Here's how the part is built. I have some questions about the finished solid (model axes, mm). A direction names the side the tool comes from. Round coordinates to 2 decimals unless told otherwise and drop trailing zeros. Write each loop counter-clockwise with the first axis right and the second up, starting at its lowest first coordinate (ties: lowest second). Pieces come first, ordered by that corner, then holes. Notation, with made-up numbers: (5.25, -21.5) - (43.25, -21.5) arc R20 ccw to (43.25, -11.5) - close; hole circle Ø7 at (40, 29). An arc over 180 degrees is marked (long way). Write item = value, one per line. Start each with the question number.
Item 1: If we section it at D-D (z = -11.25): Give the number of separate pieces and of enclosed holes in the cut face, and give its area (3 significant figures).
Item 2: If we section it at C-C (y = 16): Please give me the cut outline in (x, z).
Item 3: Thinking about a two-plate mould opening in Y: for faces 1 (the face through (-13, 66, -4)), 2 (the face through (-43, 8, -1)), 3 (the face through (-54.464, 4.056, -1.122)), 4 (the face through (-13, 0, -4)), which applies, pulls with the +Y half, pulls with the -Y half, needs draft (parallel to the pull), parting line crosses it, or undercut?
Item 4: Which directions (+Z, -Z, +X, -X, +Y, -Y) give clear straight access to the entire face, cutting with the end or side of a thin tool? Please do faces 5 (the face through (-23, 26, -5.797)), 6 (the face through (21.389, 61.944, -7.425)), 7 (the face through (-23.5, 41, -0.9)).
Item 5: If we section it at A-A (x = -53): Please give me the cut outline in (y, z), and give its area (3 significant figures).
Item 6: If we section it at B-B (x = -39.5): Please give me the cut outline in (y, z).
Item 7: For P1, Ø2.5, axis at x = -25.79, z = -0.8, coming from the -Y side; P2, Ø5, axis at x = -41, z = -8, coming from the +Y side; P3, Ø8, axis at y = 50, z = -2.5, coming from the -X side; P4, Ø3, axis at y = 39, z = -6.5, coming from the -X side, each with a flat end and sliding along its axis, tell me the tip position at first contact or that it passes through.
Item 8: If I drill on line 1 along Y through (x, z) = (-30, -1.5); line 2 along Y through (x, z) = (-41, 3.25); line 3 along Z through (x, y) = (-21, 27), over which ranges is the centre line in solid material (lowest first)? Write a range as [from, to].
```python
from build123d import *

# Parameters (mm, degrees)
BOSS_EXTRUDE1_DEPTH = 8
SKETCH2_R           = 1.7
SKETCH2_R_2         = 1.5
CUT_EXTRUDE1_DEPTH  = 10
FILLET1_SIZE        = 5
SKETCH3_R           = 5
BOSS_EXTRUDE2_DEPTH = 22
SKETCH4_R           = 1.7
CUT_EXTRUDE2_DEPTH  = 74.393131138
BOSS_EXTRUDE4_DEPTH = 22
SKETCH9_R           = 1.7
CUT_EXTRUDE3_DEPTH  = 17
SKETCH10_W          = 5
SKETCH10_H          = 10
BOSS_EXTRUDE5_DEPTH = 3


with BuildPart() as part:
    # Sketch1 → Boss-Extrude1 (new body)
    with BuildSketch(Plane(origin=(0, 0, 0), x_dir=(1, 0, 0), z_dir=(0, 1, 0))):
        Polygon((0, 5.796570021), (-65, 5.796570021), (-65, -4.203429979), (0, -4.203429979), (42, 8.002969552), (39.5, 17.276398151), align=None)
    extrude(amount=BOSS_EXTRUDE1_DEPTH)

    # Sketch2 → Cut-Extrude1 (cut)
    with BuildSketch(Plane(origin=(0, 8, 0), x_dir=(1, 0, 0), z_dir=(0, 1, 0))):
        with Locations(Location((-59, 0.796570021, 0), (0, 0, 270))):
            Circle(SKETCH2_R)
        with Locations(Location((-53, 0.796570021, 0), (0, 0, 270))):
            Circle(SKETCH2_R_2)
        with Locations(Location((-35.792921067, 0.796570021, 0), (0, 0, 270))):
            Circle(SKETCH2_R_2)
        with Locations(Location((20.375, 6.319841926, 0), (0, 0, 270))):
            Circle(SKETCH2_R_2)
        with Locations(Location((35.015323176, 10.860923065, 0), (0, 0, 270))):
            Circle(SKETCH2_R)
        with Locations(Location((0, 0.796570021, 0), (0, 0, 270))):
            Circle(SKETCH2_R_2)
    extrude(amount=-CUT_EXTRUDE1_DEPTH, mode=Mode.SUBTRACT)

    # Fillet1
    # a fillet whose section is not a circle: 5 mm, written as the material it takes off along each edge
    with BuildSketch(Plane(origin=(-65, -12.5, 4.203429979), x_dir=(0, 0, -1), z_dir=(0, 1, 0)), Plane(origin=(-65, -12.5, -5.796570021), x_dir=(1, 0, 0), z_dir=(0, 1, 0))) as fillet1_piece_1:
        with BuildLine():
            Bezier((FILLET1_SIZE, 0), (0, 0), (0, -FILLET1_SIZE), weights=[1, 1, 1])
            Line((0, -FILLET1_SIZE), (0, 0))
            Line((0, 0), (FILLET1_SIZE, 0))
        make_face()
    extrude(amount=33, mode=Mode.SUBTRACT)

    # Fillet2
    # a fillet whose section is not a circle: 5 mm, written as the material it takes off along each edge
    with BuildSketch(Plane(origin=(39.5, -12.746283343, -17.276398151), x_dir=(-0.9602675163397548, 0, 0.27908116572545455), z_dir=(0, 1, 0))) as fillet2_piece_1:
        with BuildLine():
            Bezier((5.098513337, 0), (0, 0), (0.099464892, 5.097543034), weights=[1, 1, 1])
            Line((0.099464892, 5.097543034), (0, 0))
            Line((0, 0), (5.098513337, 0))
        make_face()
    extrude(amount=33.492566686, mode=Mode.SUBTRACT)
    with BuildSketch(Plane(origin=(42, -12.258475337, -8.002969552), x_dir=(-0.2602945720874772, 0, -0.9655292516241013), z_dir=(0, 1, 0))) as fillet2_piece_2:
        with BuildLine():
            Bezier((4.903390135, 0), (0, 0), (-0.09565831, 4.902456966), weights=[1, 1, 1])
            Line((-0.09565831, 4.902456966), (0, 0))
            Line((0, 0), (4.903390135, 0))
        make_face()
    extrude(amount=32.516950674, mode=Mode.SUBTRACT)

    # Sketch3 → Boss-Extrude2 (add)
    with BuildSketch(Plane(origin=(0, 8, 0), x_dir=(1, 0, 0), z_dir=(0, 1, 0))):
        with Locations(Location((-25.792921067, 0.796570021, 0), (0, 0, 270))):
            Circle(SKETCH3_R)
    extrude(amount=BOSS_EXTRUDE2_DEPTH)

    # Sketch4 → Cut-Extrude2 (cut, through all)
    with BuildSketch(Plane(origin=(0, 30, 0), x_dir=(1, 0, 0), z_dir=(0, 1, 0))):
        with Locations(Location((-25.792921067, 0.796570021, 0), (0, 0, 270))):
            Circle(SKETCH4_R)
    extrude(amount=-CUT_EXTRUDE2_DEPTH, mode=Mode.SUBTRACT)

    # Sketch6 → Boss-Extrude4 (add)
    with BuildSketch(Plane(origin=(0, 8, 0), x_dir=(1, 0, 0), z_dir=(0, 1, 0))):
        with BuildLine():
            Line((-15.792921067, 5.796570021), (-25.792921067, 5.796570021))
            ThreePointArc((-25.792921067, 5.796570021), (-20.792921067, 0.796570021), (-25.792921067, -4.203429979))
            Line((-25.792921067, -4.203429979), (-15.792921067, -4.203429979))
            Line((-15.792921067, -4.203429979), (-15.792921067, 5.796570021))
        make_face()
    extrude(amount=BOSS_EXTRUDE4_DEPTH)

    # Sketch9 → Cut-Extrude3 (cut)
    with BuildSketch(Plane(origin=(0, 25, 0), x_dir=(1, 0, 0), z_dir=(0, 1, 0))):
        with BuildLine():
            Line((-25.792921067, 5.796570021), (-20.792921067, 5.796570021))
            Line((-20.792921067, 5.796570021), (-20.792921067, -4.203429979))
            Line((-20.792921067, -4.203429979), (-25.792921067, -4.203429979))
            ThreePointArc((-25.792921067, -4.203429979), (-30.792921067, 0.796570021), (-25.792921067, 5.796570021))
        make_face()
        with Locations(Location((-25.792921067, 0.796570021, 0), (0, 0, 270))):
            Circle(SKETCH9_R, mode=Mode.SUBTRACT)
    extrude(amount=-CUT_EXTRUDE3_DEPTH, mode=Mode.SUBTRACT)

    # Sketch10 → Boss-Extrude5 (add)
    with BuildSketch(Plane(origin=(0, 30, 0), x_dir=(1, 0, 0), z_dir=(0, 1, 0))):
        with Locations((-18.292921067, 0.796570021)):
            Rectangle(SKETCH10_W, SKETCH10_H)
    extrude(amount=BOSS_EXTRUDE5_DEPTH)

    # Mirror1: part across plane


with BuildPart() as part_1:
    add(part.part)
    add(part.part.mirror(Plane.ZX.offset(33)))


solid = part_1.part
```
Reply:
q1.separate_pieces = 4
q1.enclosed_holes = 0
q1.area = 303 mm2
q2.outline = (-20.79, -5.8) - (-15.79, -5.8) - (-15.79, 4.2) - (-20.79, 4.2) - close
q3.face_1 = pulls with the +Y half
q3.face_2 = undercut
q3.face_3 = needs draft
q3.face_4 = pulls with the -Y half
q4.face_5 = -Z, -X, +Y, -Y
q4.face_6 = +Y, -Y
q4.face_7 = +Z, -Z, -X
q5.outline = (0, -5.8) - (8, -5.8) - (8, -2.3) - (0, -2.3) - close; (0, 0.7) - (8, 0.7) - (8, 4.2) - (0, 4.2) - close; (58, -5.8) - (66, -5.8) - (66, -2.3) - (58, -2.3) - close; (58, 0.7) - (66, 0.7) - (66, 4.2) - (58, 4.2) - close
q5.area = 112 mm2
q6.outline = (0, -5.8) - (8, -5.8) - (8, 4.2) - (0, 4.2) - close; (58, -5.8) - (66, -5.8) - (66, 4.2) - (58, 4.2) - close
q7.P1 = through
q7.P2 = 66
q7.P3 = -20.79
q7.P4 = -28.5
q8.line_1 = [0, 8], [25, 30], [36, 41], [58, 66]
q8.line_2 = [0, 8], [58, 66]
q8.line_3 = [-5.8, 4.2]
